Autodesk Inventor part; units mm, degrees
ref_plane "Work Plane1" through (7.5, 0, 0) normal (0, 0.5, 0.8660254) x (1, 0, 0)
ref_plane "YZ Plane" through (0, 0, 0) normal (1, 0, 0) x (0, 1, 0)
ref_plane "XZ Plane" through (0, 0, 0) normal (0, 1, 0) x (-1, 0, 0)
sketch "草圖1" plane through (0, 0, 0) normal (0, 0, 1) x (1, 0, 0)
  line L0 (1.2217, 0) -> (15, 0)
  line L1 (15, 0) -> (15, 2.5)
  line L2 (15, 2.5) -> (0, 2.5)
  line L3 (0, 2.5) -> (0, 4.25)
  line L4 (0, 4.25) -> (-3.5, 4.25)
  line L5 (-3.5, 4.25) -> (-3.5, 2.3094)
  line L6 (-3.5, 2.3094) -> (-1.5, 2.3094)
  line L7 (-1.5, 2.3094) -> (-0.8884, 1.25)
  line L8 (-7.2, 0) -> (18.7, 0)
  line L9 (0, -0.85) -> (0, 5.1)
  line L10 (-0.8884, 1.25) -> (0.5, 1.25)
  line L11 (0.5, 1.25) -> (1.2217, 0)
  line L12 (-3.5, 2.3094) -> (-3.5, 0) construction
  dimension "d0" = 3.5
  dimension "d1" = 2
  dimension "d2" = 60
  dimension "d3" = 5
  dimension "d4" = 4.6188
  dimension "d5" = 8.5
  dimension "d15" = 4
  dimension "d16" = 2.5
  dimension "d17" = 15
revolve "本體" add sketch "草圖1" angle 360 about axis through (1.2217, 0, 0) along (1, 0, 0) contours L11 L10 L9 L2 L1 L0 | L10 L7 L6 L5 L4 L3 L9
sketch "草圖2" plane through (-3.5, 0, 0) normal (-1, 0, 0) x (0, 0, 1)
  circle A0 centre (0, 0) radius 2.3094
  line L0 (0, -5.95) -> (0, 5.95)
  line L1 (-5.95, 0) -> (5.95, 0)
  line L2 (2.3094, 0) -> (1.1547, -2)
  line L3 (1.1547, -2) -> (-1.1547, -2)
  line L4 (-1.1547, -2) -> (-2.3094, 0)
  line L5 (-2.3094, 0) -> (-1.1547, 2)
  line L6 (-1.1547, 2) -> (1.1547, 2)
  line L7 (1.1547, 2) -> (2.3094, 0)
extrude "塞槽" add sketch "草圖2" against normal up to next contours L7 A0 | A0 L2 | L6 L0 A0 | A0 L0 L3 | L0 L6 A0 | A0 L3 L0 | L4 A0 | A0 L5
thread "螺紋"
chamfer "倒角1" distance 0.4908 distance2 0.4908 1 edges at (15, -2.5, 0) measured on face at (15, -0.7741, -0.6858)
ref_plane "Work Plane1" through (7.5, 0, 0) normal (0, 0.5, 0.8660254) x (1, 0, 0)
equation "\"d7\" = GEL"
equation "\"d9\" = -0.5 * SPD + 0.5 * GD"
equation "\"d12\" = GUL"
equation "\"d0\" = KOH"
equation "\"d1\" = INTI"
equation "\"d3\" = GD"
equation "\"d4\" = 1.1547 * SW"
equation "\"d5\" = KOD"
equation "\"d15\" = INFT"
equation "\"d16\" = SDT"
equation "\"d17\" = NLG"
equation "\"GD\" = NND"
equation "\"NLG\" = 15"
equation "\"GEL\" = 12.4"
equation "\"KOD\" = 8.5"
equation "\"KOH\" = 3.5"
equation "\"GUL\" = 0.61345 * PTC"
equation "\"SW\" = 4"
equation "\"INTI\" = 2"
equation "\"SPD\" = NND - 1.2269 * PTC"
equation "\"SDT\" = 2.5"
equation "\"INFT\" = 4"
equation "\"TOA\" = 30deg"
equation "\"GD1\" = THREADDIA - 1.2269 * PTC"
equation "\"THREADDIA\" = 5"
equation "\"BDM\" = NND"
equation "\"RR\" = 0.5"
equation "\"PTC\" = 0.8"
equation "\"NND\" = 5"
equation "\"SLG\" = 2.6"
equation "\"GAL\" = 0.61345 * PTC"
equation "\"E0\" = 1.155 * SW"
properties part number "CNS 4557 - M5 x 15" material "鋼、軟鋼"
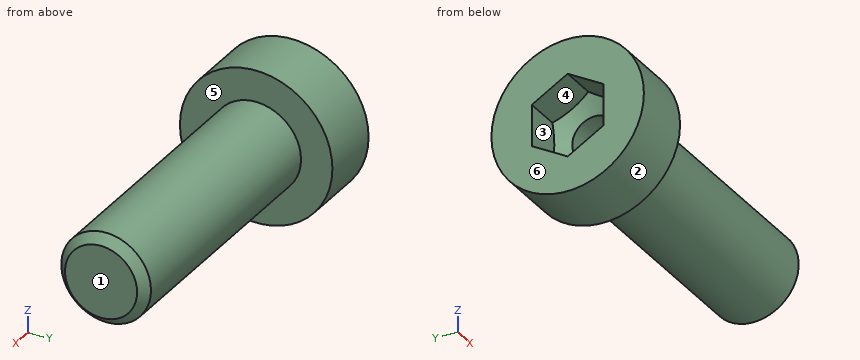
Check sheet for the modelled part. Datum: model origin and axes. Units: mm. Face numbers are marked on the shaded views. A direction names the side the tool comes from. Round coordinates to 2 decimals unless told otherwise and drop trailing zeros. Write each loop counter-clockwise with the first axis right and the second up, starting at its lowest first coordinate (ties: lowest second). Pieces come first, ordered by that corner, then holes. Notation, with made-up numbers: (-4.5, -1) -> (42.5, -1) arc R10 ccw to (42.5, 10) -> close; hole circle Ø8 at (59, 28). An arc over 180 degrees is marked (long way). Answer as CSV lines item,"result". Start each with the question number.
1) Release check for a two-part mould opening along Z. For the marked faces 1, 2 and 3 record: pulls with the +Z half, pulls with the -Z half, needs draft (parallel to the pull), parting line crosses it, or undercut.
2) Section check C-C on y = 3. Enter the section's corners in (x, z), and give its area (3 significant figures).
3) Section check A-A on z = 3.75. Enter the section's corners in (x, y), and give its area (3 significant figures).
4) Go/stop test with flat-tipped pins: P1, Ø1.1, axis at x = -2, z = 0.5, coming from the +Y side; P2, Ø1.5, axis at x = 6.5, y = 0.5, coming from the -Z side; P3, Ø1.5, axis at x = 1, y = 0, coming from the +Z side; P4, Ø2, axis at x = 0, y = 2, coming from the -Z side. Record where each tip stops, or that it passes through.
5) Tool access check on the marked faces 4, 5 and 6. Record the directions out of +Z, -Z, +X, -X, +Y, -Y that give a thin tool (end or side, any length) a straight path to the whole face; none if there is none.
6) Section check B-B on x = 14. Enter the section's corners in (y, z).
7) Material ranges on line 1 (Z direction, x = 0.05, y = 0); line 2 (Z direction, x = 12.5, y = -1.5); line 3 (X direction, y = 2.75, z = -2.25), recorded low to high. Write a range as from..to.
Found:
1,face 1,"needs draft"
1,face 2,"parting line crosses it"
1,face 3,"undercut"
2,outline,"(-3.5, -3.01) -> (0, -3.01) -> (0, 3.01) -> (-3.5, 3.01) -> close"
2,area,"21.1 mm^2"
3,outline,"(-3.5, -2) -> (0, -2) -> (0, 2) -> (-3.5, 2) -> close"
3,area,"14.0 mm^2"
4,P1,"stops at y = 4.25"
4,P2,"stops at z = -2.5"
4,P3,"stops at z = 2.5"
4,P4,"stops at z = -4.13"
5,face 4,"-X"
5,face 5,"+X"
5,face 6,"+Z, -Z, -X, +Y, -Y"
6,outline,"circle Ø5 at (0, 0)"
7,line 1,"z = -2.5..-1.25, 1.25..2.5"
7,line 2,"z = -2..2"
7,line 3,"x = -3.5..0"
